```python
from build123d import *

# Parameters (mm, degrees)
F0_W     = 45
F0_H     = 37
F1_DEPTH = 8
F3_DEPTH = 37.001
F4_W     = 45.155443
F4_H     = 1.4
F4_W_2   = 45.195
F4_H_2   = 2.4
F5_DEPTH = 37.001
F6_W     = 32
F6_H     = 32
F7_DEPTH = 1.601


with BuildPart() as f1:
    # F0 (on Top) → F1 (new body)
    with BuildSketch(Plane.XY):
        Rectangle(F0_W, F0_H)
    extrude(amount=F1_DEPTH)

    # F2 (on face) → F3 (cut, through all)
    with BuildSketch(Plane.XZ.offset(18.5)):
        Polygon((15.7, 8), (-15.7, 8), (-17.7, 3.392867), (-17.7, 3), (17.7, 3), (17.7, 3.392867), align=None)
    extrude(amount=-F3_DEPTH, mode=Mode.SUBTRACT)

    # F4 (on face) → F5 (cut, through all)
    with BuildSketch(Plane.XZ.offset(18.5)):
        with Locations((0.003687, 0.7)):
            Rectangle(F4_W, F4_H)
        with Locations((0.023347, 6.901389)):
            Rectangle(F4_W_2, F4_H_2)
    extrude(amount=-F5_DEPTH, mode=Mode.SUBTRACT)

    # F6 (on face) → F7 (cut, through all)
    with BuildSketch(Plane.XY.offset(3)):
        Rectangle(F6_W, F6_H)
    extrude(amount=-F7_DEPTH, mode=Mode.SUBTRACT)


solid = f1.part
```
Geometry check sheet. Reference: the model listing, model coordinates, mm. A direction names the side the tool comes from. Coordinates: 2 decimals unless noted, no trailing zeros. Write each loop counter-clockwise with the first axis right and the second up, starting at its lowest first coordinate (ties: lowest second). Pieces come first, ordered by that corner, then holes. Notation, with made-up numbers: M 26.25,-6 L 60.25,-6 A10 ccw 60.25,0 Z; hole C 60,48 d9. An arc over 180 degrees is marked long. Use one line per item in the form item = value. Start each with the question number.
1) Release check for a two-part mould opening along X. For faces 4 (the flat face through (17.206, -0.259, 4.531)), 5 (the flat face through (22.5, 0, 4)), 6 (the flat face through (-22.5, 0, 4)) record: pulls with the +X half, pulls with the -X half, needs draft (parallel to the pull), parting line crosses it, or undercut.
2) Thickness scan on probe 1 along Y at (x, z) = (-2, 2.45); probe 2 along X at (y, z) = (-2, 2.85); probe 3 along X at (y, z) = (0, 3.6). Record the ranges inside material, lowest first. Write a range as from..to.
3) Section check B-B on x = -11. Enter the section's corners in (y, z).
4) Section check C-C on z = 4.8. Enter the section's corners in (x, y), and give its area (3 significant figures).
5) Set-up check for faces 1 (the flat face through (0, 16, 2)), 2 (the flat face through (-0.3, 18.5, 2.6)), 3 (the flat face through (-17.192, -0.259, 4.563)): record each of +Z, -Z, +X, -X, +Y, -Y from which the full face is reachable in a straight line by a thin tool's end or side.
6) Section check A-A on y = -12. Enter the section's corners in (x, z).
Responses:
q1.face_4 = undercut
q1.face_5 = pulls with the +X half
q1.face_6 = pulls with the -X half
q2.probe_1 = -18.5..-16, 16..18.5
q2.probe_2 = -22.5..-16, 16..22.5
q2.probe_3 = -22.5..-17.61, 17.61..22.5
q3.outline = M -18.5,1.4 L -16,1.4 L -16,3 L -18.5,3 Z; M 16,1.4 L 18.5,1.4 L 18.5,3 L 16,3 Z
q4.outline = M -22.5,-18.5 L -17.09,-18.5 L -17.09,18.5 L -22.5,18.5 Z; M 17.09,-18.5 L 22.5,-18.5 L 22.5,18.5 L 17.09,18.5 Z
q4.area = 400 mm2
q5.face_1 = +Z, -Z
q5.face_2 = +Z, -Z, +X, -X, +Y
q5.face_3 = +Y, -Y
q6.outline = M -22.5,1.4 L -16,1.4 L -16,3 L -17.7,3 L -17.7,3.39 L -16.7,5.7 L -22.5,5.7 Z; M 16,1.4 L 22.5,1.4 L 22.5,5.7 L 16.7,5.7 L 17.7,3.39 L 17.7,3 L 16,3 Z
